from build123d import *

# Parameters (mm, degrees)
SKETCH1_R           = 11
SKETCH1_R_2         = 6.5
BOSS_EXTRUDE1_DEPTH = 5
BOSS_EXTRUDE2_START = 5
SKETCH1_3_R         = 13
SKETCH1_3_R_2       = 11
BOSS_EXTRUDE2_DEPTH = 3.5
BOSS_EXTRUDE3_START = -5
SKETCH1_5_R         = 6.5
SKETCH1_5_R_2       = 2.5
BOSS_EXTRUDE3_DEPTH = 5
BOSS_EXTRUDE4_START = -1.5
SKETCH1_6_R         = 13
SKETCH1_6_R_2       = 11
BOSS_EXTRUDE4_DEPTH = 3.5


with BuildPart() as part:
    # Sketch1 → Boss-Extrude1 (new, symmetric)
    with BuildSketch(Plane.XY):
        Circle(SKETCH1_R)
        Circle(SKETCH1_R_2, mode=Mode.SUBTRACT)
    extrude(amount=BOSS_EXTRUDE1_DEPTH, both=True)

    # Sketch1<3> → Boss-Extrude2 (add)
    with BuildSketch(Plane.XY.offset(BOSS_EXTRUDE2_START)):
        Circle(SKETCH1_3_R)
        Circle(SKETCH1_3_R_2, mode=Mode.SUBTRACT)
    extrude(amount=-BOSS_EXTRUDE2_DEPTH)

    # Sketch1<5> → Boss-Extrude3 (add)
    with BuildSketch(Plane.XY.offset(BOSS_EXTRUDE3_START)):
        Circle(SKETCH1_5_R)
        Circle(SKETCH1_5_R_2, mode=Mode.SUBTRACT)
    extrude(amount=BOSS_EXTRUDE3_DEPTH)

    # Sketch1<6> → Boss-Extrude4 (add)
    with BuildSketch(Plane.XY.offset(BOSS_EXTRUDE4_START)):
        Circle(SKETCH1_6_R)
        Circle(SKETCH1_6_R_2, mode=Mode.SUBTRACT)
    extrude(amount=-BOSS_EXTRUDE4_DEPTH)


solid = part.part
The listing builds one solid part. Answer for the finished solid, in the listing's coordinates (mm). A direction names the side the tool comes from. Round coordinates to 2 decimals unless told otherwise and drop trailing zeros. Order: outer loops, then holes, each group sorted by start corner. A loop starts at its lowest first (then second) coordinate and runs counter-clockwise, first axis right, second up. Notation, with made-up numbers: (43, 87.5) -> (57, 87.5) arc R25 cw to (57, 112.5) -> close; hole circle Ø3 at (-0.75, 26.25). An arc over 180 degrees is marked (long way). One line per item, written item: value.
Item 1: For faces 1 (the flat face through (-11, 3, -1.5)), 2 (the cylindrical face through (-0.54, -2.44, -2.54)), 3 (the cylindrical face through (-5.158, -3.955, 2.465)), determine the directions among +Z, -Z, +X, -X, +Y, -Y from which every point of the face is accessible in a straight line to the end or side of a thin tool.
Taken from the geometry:
face 1: none
face 2: +Z, -Z
face 3: +Z
Item 2: Given P1, Ø6, axis at y = 8.5, z = -0.5, coming from the -X side; P2, Ø5, axis at x = -10, z = -1.5, coming from the +Y side; P3, Ø3, axis at x = -4.5, z = -1, coming from the +Y side, each flat-ended and moving along its own axis, determine where each tip first touches the part or whether it passes through.
Taken from the geometry:
P1: stops at x = -11.7
P2: stops at y = 10.62
P3: stops at y = 12.63
Item 3: For a pull along Y with two mould halves and no side action, classify faces 4 (the flat face through (-11, 3, 1.5)), 5 (the cylindrical face through (-10.316, -7.91, 3.274)), 6 (the flat face through (3, 0, 0)) as released by +Y, released by -Y, zero draft, split by the parting line, or undercut.
Taken from the geometry:
face 4: zero draft
face 5: split by the parting line
face 6: undercut
Item 4: Find section A-A, the plane x = 0. Give the vertices of the cut face in (y, z).
Taken from the geometry:
outline: (-13, -5) -> (-2.5, -5) -> (-2.5, 0) -> (-6.5, 0) -> (-6.5, 5) -> (-13, 5) -> (-13, 1.5) -> (-11, 1.5) -> (-11, -1.5) -> (-13, -1.5) -> close; (2.5, -5) -> (13, -5) -> (13, -1.5) -> (11, -1.5) -> (11, 1.5) -> (13, 1.5) -> (13, 5) -> (6.5, 5) -> (6.5, 0) -> (2.5, 0) -> close
Item 5: Find section C-C, the plane z = -2.5. Give the vertices of the cut face in (x, y).
Taken from the geometry:
outline: circle Ø26 at (0, 0); hole circle Ø5 at (0, 0)
Item 6: Straight lines are drawn through the part: L1, parallel to Z at x = 4.5, y = -10.75; L2, parallel to Y at x = 0, z = -1.75; L3, parallel to Y at x = 0, z = 2.75. For each, find the intervals that lie inside material, in ascending order.
Taken from the geometry:
L1: z = -5 to -1.5, 1.5 to 5
L2: y = -13 to -2.5, 2.5 to 13
L3: y = -13 to -6.5, 6.5 to 13
Item 7: Find section D-D, the plane y = -7.25. Give the vertices of the cut face in (x, z), then the cut area to 3 significant figures.
Taken from the geometry:
outline: (-10.79, -5) -> (10.79, -5) -> (10.79, -1.5) -> (8.27, -1.5) -> (8.27, 1.5) -> (10.79, 1.5) -> (10.79, 5) -> (-10.79, 5) -> (-10.79, 1.5) -> (-8.27, 1.5) -> (-8.27, -1.5) -> (-10.79, -1.5) -> close
area: 201 mm2
